Can you work these out from the drawing? Everything is in mm from the part's minimum corner. A direction names the side the tool comes from. Round coordinates to 2 decimals unless told otherwise and drop trailing zeros. Order: outer loops, then holes, each group sorted by start corner. A loop starts at its lowest first (then second) coordinate and runs counter-clockwise, first axis right, second up. Notation, with made-up numbers: (2, 38) - (49, 38) arc R26 cw to (49, 52) - close; hole circle Ø8 at (82, -33). An arc over 180 degrees is marked (long way). Answer as a JSON object with one key per item and string values.
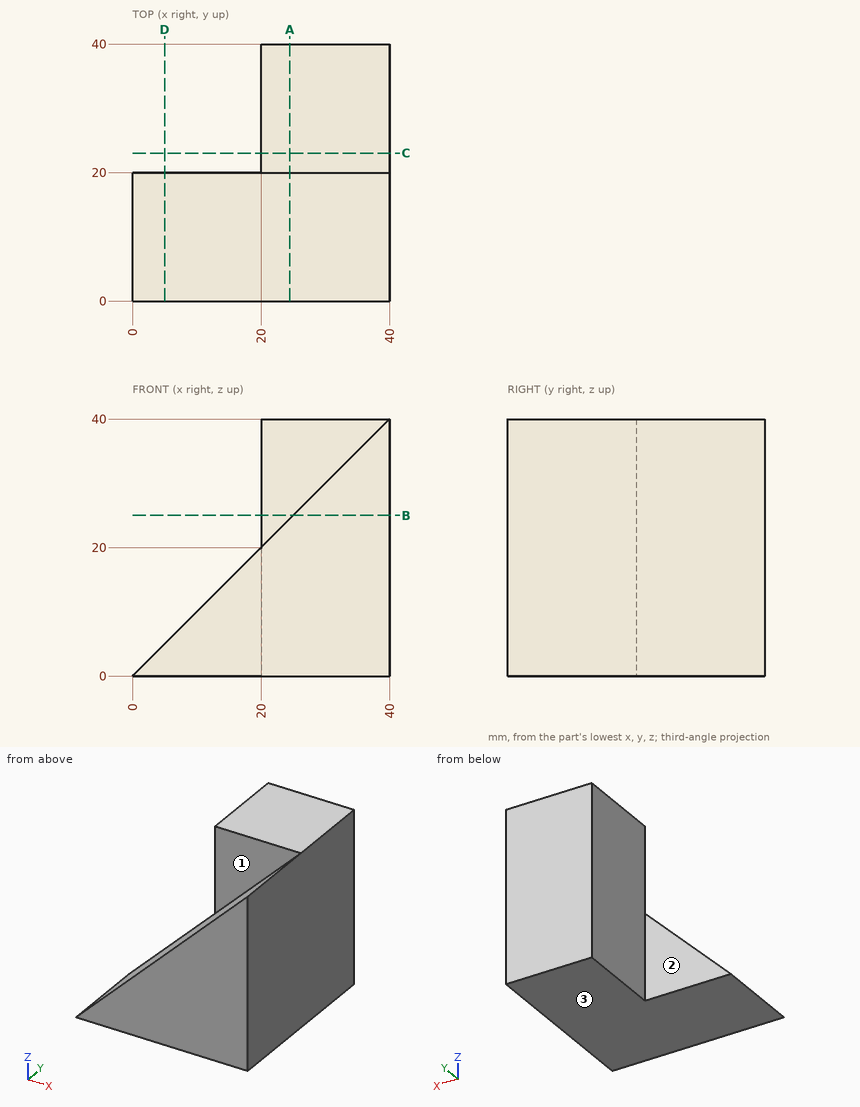
1. For P1, Ø6, axis at y = 12.5, z = 35, coming from the -X side; P2, Ø10, axis at x = 7.5, z = 14.5, coming from the +Y side; P3, Ø6, axis at y = 32, z = 20, coming from the -X side; P4, Ø10, axis at x = 28, z = 33.5, coming from the -Y side, each with a flat end and sliding along its axis, tell me the tip position at first contact or that it passes through.
Responses:
{"P1": "x = 32", "P2": "y = 20", "P3": "x = 20", "P4": "y = 0"}
2. If I drill on L1, parallel to X at y = 28, z = 6; L2, parallel to Z at x = 38.5, y = 12.5; L3, parallel to Z at x = 34.5, y = 6, over which ranges is the centre line in solid material (lowest first)? Write a range as [from, to].
Responses:
{"L1": "[20, 40]", "L2": "[0, 38.5]", "L3": "[0, 34.5]"}
3. For the marked faces 1, 2 and 3, which set-ups out of +Z, -Z, +X, -X, +Y, -Y let a thin tool reach every point of the face, with its end or its side?
Responses:
{"face 1": "+Z, -X, -Y", "face 2": "+Z, -Z, -X, +Y", "face 3": "-Z, +X, -X, +Y, -Y"}
4. Imagine slicing it at C-C (y = 23). List the corners of the cut face in (x, z) for me, plus the area to 3 significant figures.
Responses:
{"outline": "(20, 0) - (40, 0) - (40, 40) - (20, 40) - close", "area": "800 mm2"}
5. Imagine slicing it at B-B (z = 25). List the corners of the cut face in (x, y) for me, plus the area to 3 significant figures.
Responses:
{"outline": "(20, 20) - (25, 20) - (25, 0) - (40, 0) - (40, 40) - (20, 40) - close", "area": "700 mm2"}
6. Imagine slicing it at A-A (x = 24.5). List the corners of the cut face in (y, z) for me.
Responses:
{"outline": "(0, 0) - (40, 0) - (40, 40) - (20, 40) - (20, 24.5) - (0, 24.5) - close"}
7. Imagine slicing it at D-D (x = 5). List the corners of the cut face in (y, z) for me, plus the area to 3 significant figures.
Responses:
{"outline": "(0, 0) - (20, 0) - (20, 5) - (0, 5) - close", "area": "100 mm2"}
